Part model, mm, in its own coordinate system. A direction names the side the tool comes from. Round coordinates to 2 decimals unless told otherwise and drop trailing zeros. Order: outer loops, then holes, each group sorted by start corner. A loop starts at its lowest first (then second) coordinate and runs counter-clockwise, first axis right, second up. Notation, with made-up numbers: (22, -27) -> (44, -27) arc R9 cw to (44, -22) -> close; hole circle Ø4 at (-9.5, 88.25). An arc over 180 degrees is marked (long way). Use CSV: the item, a comma, the result in double quotes.
Autodesk Inventor part; units mm, degrees
ref_plane "YZ Plane" through (0, 0, 0) normal (1, 0, 0) x (0, 1, 0)
ref_plane "XZ Plane" through (0, 0, 0) normal (0, 1, 0) x (-1, 0, 0)
ref_plane "XY Plane" through (0, 0, 0) normal (0, 0, 1) x (1, 0, 0)
sketch "Эскиз1" plane through (0, 0, 0) normal (0, 0, 1) x (1, 0, 0)
  line L0 (25, -17.5) -> (-25, -17.5)
  line L1 (-25, -17.5) -> (-25, 17.5)
  line L2 (-25, 17.5) -> (25, 17.5)
  line L3 (25, 17.5) -> (25, -17.5)
  line L4 (25, -17.5) -> (-25, 17.5) construction
  line L5 (-25, -17.5) -> (25, 17.5) construction
  line L6 (-25, 17.5) -> (-10, 17.5)
  line L7 (-10, 17.5) -> (-10, 23.5)
  line L8 (-10, 23.5) -> (-25, 23.5)
  line L9 (-25, 23.5) -> (-25, 17.5)
  line L10 (25, 17.5) -> (10, 17.5)
  line L11 (10, 17.5) -> (10, 23.5)
  line L12 (10, 23.5) -> (25, 23.5)
  line L13 (25, 23.5) -> (25, 17.5)
  line L14 (-25, -17.5) -> (-10, -17.5)
  line L15 (-10, -17.5) -> (-10, -23.5)
  line L16 (-10, -23.5) -> (-25, -23.5)
  line L17 (-25, -23.5) -> (-25, -17.5)
  line L18 (25, -17.5) -> (10, -17.5)
  line L19 (10, -17.5) -> (10, -23.5)
  line L20 (10, -23.5) -> (25, -23.5)
  line L21 (25, -23.5) -> (25, -17.5)
  line L22 (0, 0) -> (0, 45.655) construction
  point P0 (-10, -17.5)
  point P1 (10, 17.5)
  dimension "d0" = 50
  dimension "d1" = 35
  dimension "d2" = 6
  dimension "d3" = 15
extrude "Выдавливание1" add sketch "Эскиз1" along normal mid plane 6
properties part number "Стойка_В5" material "По умолчанию1"
(1) Which spindle directions (+Z, -Z, +X, -X, +Y, -Y) get a long thin tool onto all of the face, cutting with end or side? Do faces 1 (the face through (25, 0, 0)), 2 (the face through (-10, 20, 0)), 3 (the face through (0, -17.5, 0)). Say none if no direction does.
Reply:
face 1,"+Z, -Z, +X, +Y, -Y"
face 2,"+Z, -Z, +Y"
face 3,"+Z, -Z, -Y"
(2) Cut at A-A, the plane y = 18.5. Give the cut face in (x, z).
Reply:
outline,"(-25, -3) -> (-10, -3) -> (-10, 3) -> (-25, 3) -> close; (10, -3) -> (25, -3) -> (25, 3) -> (10, 3) -> close"
(3) Probe probe 1 along X at (y, z) = (18, 0.8); probe 2 along Y at (x, z) = (8, 2.75). List the from-to ranges inside material, lowest first. Write a range as [from, to].
Reply:
probe 1,"[-25, -10], [10, 25]"
probe 2,"[-17.5, 17.5]"
(4) Drop flat-ended pins along their axis: P1, Ø3, axis at x = -2, z = 0, coming from the +Y side; P2, Ø1.8, axis at x = -3, z = -1, coming from the -Y side. Give the stop position or say it passes through.
Reply:
P1,"y = 17.5"
P2,"y = -17.5"
(5) Cut at C-C, the plane x = 1. Give the cut face in (y, z), then the cut area to 3 significant figures.
Reply:
outline,"(-17.5, -3) -> (17.5, -3) -> (17.5, 3) -> (-17.5, 3) -> close"
area,"210 mm2"
(6) Pull direction X, two halves, no side cores. Call faces 4 (the face through (-17, -23.5, 0)), 5 (the face through (0, 17.5, 0)), 6 (the face through (-25, 0, 0)): released by +X, released by -X, zero draft, split by the parting line, or undercut.
Reply:
face 4,"zero draft"
face 5,"undercut"
face 6,"released by -X"
(7) Cut at B-B, the plane z = 0.2. Give the cut face in (x, y), then the cut area to 3 significant figures.
Reply:
outline,"(-25, -23.5) -> (-10, -23.5) -> (-10, -17.5) -> (10, -17.5) -> (10, -23.5) -> (25, -23.5) -> (25, 23.5) -> (10, 23.5) -> (10, 17.5) -> (-10, 17.5) -> (-10, 23.5) -> (-25, 23.5) -> close"
area,"2,110 mm2"
